```python
from build123d import *

# Parameters (mm, degrees)
BOSS_EXTRUDE1_DEPTH                                 = 12.7
F_4_CLEARANCE_HOLE1_D                               = 3.3
F_4_CLEARANCE_HOLE1_DEPTH                           = 12.7
F_1_4_CLEARANCE_HOLE1_D                             = 6.6
F_1_4_CLEARANCE_HOLE1_DEPTH                         = 12.7
F_1_4_CLEARANCE_HOLE2_D                             = 6.8
F_1_4_CLEARANCE_HOLE2_DEPTH                         = 12.7
CSK_FOR_1_4_FLAT_HEAD_MACHINE_SCREW_100_D           = 6.6
CSK_FOR_1_4_FLAT_HEAD_MACHINE_SCREW_100_DEPTH       = 12.7
CSK_FOR_1_4_FLAT_HEAD_MACHINE_SCREW_100_CSINK_D     = 12.6
CSK_FOR_1_4_FLAT_HEAD_MACHINE_SCREW_100_CSINK_ANGLE = 90
F_10_CLEARANCE_HOLE1_D                              = 5
F_10_CLEARANCE_HOLE1_DEPTH                          = 15
F_10_CLEARANCE_HOLE2_D                              = 5
F_10_CLEARANCE_HOLE2_DEPTH                          = 10
F_1_3_4_CLEARANCE_HOLE1_D                           = 45
F_1_3_4_CLEARANCE_HOLE1_DEPTH                       = 5
F_1_4_CLEARANCE_HOLE3_D                             = 6.6
F_1_4_CLEARANCE_HOLE3_DEPTH                         = 12.7
CHAMFER1_SIZE                                       = 3
BOSS_EXTRUDE2_DEPTH                                 = 12.7


with BuildPart() as part:
    # Sketch1 → Boss-Extrude1 (new body)
    with BuildSketch(Plane(origin=(0, 0, 0), x_dir=(-1, 0, 0), z_dir=(0, 0, -1))):
        with BuildLine():
            Line((44.45, 0), (44.45, 60))
            Line((44.45, 60), (-44.45, 60))
            Line((-44.45, 60), (-44.45, 0))
            ThreePointArc((-44.45, 0), (0, -44.45), (44.45, 0))
        make_face()
    extrude(amount=-BOSS_EXTRUDE1_DEPTH)

    # #4 Clearance Hole1
    with Locations(Plane.XY.offset(12.7)):
        with Locations((32.349998458, 0.009014041), (6, -26.35), (-20.349998115, -0.009967087), (6, 26.35)):
            Hole(F_4_CLEARANCE_HOLE1_D / 2, depth=F_4_CLEARANCE_HOLE1_DEPTH)

    # 1/4 Clearance Hole1
    with Locations(Plane(origin=(0, 0, 0), x_dir=(-1, 0, 0), z_dir=(0, 0, -1))):
        with Locations((8.85, 30), (23.65, 38), (23.65, 22)):
            Hole(F_1_4_CLEARANCE_HOLE1_D / 2, depth=F_1_4_CLEARANCE_HOLE1_DEPTH)

    # 1/4 Clearance Hole2
    with Locations(Plane.XY.offset(12.7)):
        with Locations((17.47250377, 49.692873304)):
            Hole(F_1_4_CLEARANCE_HOLE2_D / 2, depth=F_1_4_CLEARANCE_HOLE2_DEPTH)

    # CSK for 1/4 Flat Head Machine Screw (100)1
    with Locations(Plane(origin=(0, 0, 0), x_dir=(-1, 0, 0), z_dir=(0, 0, -1))):
        with Locations((23.65, 54), (38.45, 6), (38.45, 30)):
            CounterSinkHole(CSK_FOR_1_4_FLAT_HEAD_MACHINE_SCREW_100_D / 2, CSK_FOR_1_4_FLAT_HEAD_MACHINE_SCREW_100_CSINK_D / 2, depth=CSK_FOR_1_4_FLAT_HEAD_MACHINE_SCREW_100_DEPTH, counter_sink_angle=CSK_FOR_1_4_FLAT_HEAD_MACHINE_SCREW_100_CSINK_ANGLE)

    # #10 Clearance Hole1
    with Locations(Plane(origin=(0, 60, 0), x_dir=(1, 0, 0), z_dir=(0, 1, 0))):
        with Locations((-38.45, -6.35), (-8.85, -6.35)):
            Hole(F_10_CLEARANCE_HOLE1_D / 2, depth=F_10_CLEARANCE_HOLE1_DEPTH)

    # #10 Clearance Hole2
    with Locations(Plane(origin=(44.45, 0, 0), x_dir=(0, 0, -1), z_dir=(1, 0, 0))):
        with Locations((-6.35, 7), (-6.35, 53), (-6.35, 30)):
            Hole(F_10_CLEARANCE_HOLE2_D / 2, depth=F_10_CLEARANCE_HOLE2_DEPTH)

    # 1-3/4 Clearance Hole1
    with Locations(Plane(origin=(0, 0, 0), x_dir=(-1, 0, 0), z_dir=(0, 0, -1))):
        with Locations((-6, 0)):
            Hole(F_1_3_4_CLEARANCE_HOLE1_D / 2, depth=F_1_3_4_CLEARANCE_HOLE1_DEPTH)

    # 1/4 Clearance Hole3
    with Locations(Plane.XY.offset(12.7)):
        with Locations((18.374368671, 12.374368671), (23.499999956, -0.001247108), (18.374368671, -12.374368671), (6, -17.5), (-6.374368671, -12.374368671), (-11.5, 0), (-6.374368671, 12.374368671), (6, 17.5)):
            Hole(F_1_4_CLEARANCE_HOLE3_D / 2, depth=F_1_4_CLEARANCE_HOLE3_DEPTH)

    # Chamfer1
    chamfer1_edges = [part.edges().sort_by_distance(p)[0] for p in [
        (-26.95, 22, 0),
        (-26.95, 38, 0),
        (-12.15, 30, 0),
    ]]
    chamfer(chamfer1_edges, length=CHAMFER1_SIZE)

    # Sketch18 → Boss-Extrude2 (add)
    with BuildSketch(Plane(origin=(0, 0, 0), x_dir=(-1, 0, 0), z_dir=(0, 0, -1))):
        with BuildLine():
            Line((-44.45, 0), (-50.45, 0))
            ThreePointArc((-50.45, 0), (-37.430896424, -31.430896424), (-6, -44.45))
            Line((-6, -44.45), (0, -44.45))
            ThreePointArc((0, -44.45), (-31.430896424, -31.430896424), (-44.45, 0))
        make_face()
    extrude(amount=-BOSS_EXTRUDE2_DEPTH)


solid = part.part
```
Read the model definition and answer for the solid it produces. Units are mm, in the model's axes. A direction names the side the tool comes from. Round coordinates to 2 decimals unless told otherwise and drop trailing zeros. Write each loop counter-clockwise with the first axis right and the second up, starting at its lowest first coordinate (ties: lowest second). Pieces come first, ordered by that corner, then holes. Notation, with made-up numbers: M 28,74.25 L 58,74.25 A23 cw 58,112.25 Z; hole C 31,-12.75 d3. An arc over 180 degrees is marked long. One line per item, written item: value.
Q1. Flat-ended cylindrical pins translate along their axes: pin 1 Ø8.5 at (x, y) = (18.37, -12.37) entering from -Z; pin 2 Ø6.5 at (y, z) = (19.5, 5) entering from +X; pin 3 Ø8.5 at (x, y) = (-38.45, 30) entering from -Z. Find the tip coordinate at first contact, or state that the pin passes through.
Data:
pin 1: z = 5
pin 2: x = 44.45
pin 3: z = 2.05
Q2. Find section D-D on z = 10.5. Count the separate pieces of the cut face and the enclosed holes in it, plus the area to 3 significant figures.
Data:
separate pieces: 1
enclosed holes: 19
area: 8,150 mm2
Q3. Straight lines are drawn through the part: line 1 (Y direction, x = 6, z = 7.75); line 2 (Y direction, x = 40.5, z = 6.35); line 3 (X direction, y = 6, z = 9.5). For each, find the intervals that lie inside material, in ascending order. Write a range as [from, to].
Data:
line 1: [-44.45, -28], [-24.7, -20.8], [-14.2, 14.2], [20.8, 24.7], [28, 60]
line 2: [-28.03, 4.5], [9.5, 27.5], [32.5, 50.5], [55.5, 60]
line 3: [-44.45, -41.75], [-35.15, 44.45]
Q4. Find section A-A on y = -17.5. Write down the section's boundary in (x, z), plus the area to 3 significant figures.
Data:
outline: M -40.86,0 L -8.14,0 L -8.14,5 L 2.7,5 L 2.7,12.7 L -40.86,12.7 Z; M 9.3,5 L 20.14,5 L 20.14,0 L 46.86,0 L 46.86,12.7 L 9.3,12.7 Z
area: 922 mm2
Q5. Find section B-B on x = 23. Write down the section's boundary in (y, z).
Data:
outline: M -41.07,0 L -14.74,0 L -14.74,5 L -3.26,5 L -3.26,12.7 L -41.07,12.7 Z; M 3.26,5 L 14.74,5 L 14.74,0 L 60,0 L 60,12.7 L 3.26,12.7 Z
Q6. Find section C-C on x = 40. Write down the section's boundary in (y, z).
Data:
outline: M -28.63,0 L 60,0 L 60,12.7 L -28.63,12.7 Z; hole C 7,6.35 d5; hole C 30,6.35 d5; hole C 53,6.35 d5
Q7. For a pull along X with two mould halves and no side action, classify faces 4 (the cylindrical face through (19.09, -15.596, 8.796)), 5 (the cylindrical face through (39.38, 5.479, 4.366)), 6 (the flat face through (-44.45, 30, 6)), 7 (the cylindrical face through (37.775, -31.083, 6.261)) as +X half, -X half, draft (parallel to the pull), parting line (faces both ways), or undercut.
Data:
face 4: undercut
face 5: draft
face 6: -X half
face 7: +X half
Q8. Which of the six approach directions +Z, -Z, +X, -X, +Y, -Y give full straight-line access (tool end or side, diameter ignored) to faces 1 (the cylindrical face through (2.85, -16.51, 8.8)), 2 (the flat face through (34.45, 53, 6)), 3 (the cylindrical face through (-6.352, 52.395, 6.24))?
Data:
face 1: +Z, -Z
face 2: +X
face 3: +Y
